from build123d import *

# Parameters (mm, degrees)
F0_W     = 19.05
F0_H     = 50.8
F0_W_2   = 25.4
F0_H_2   = 19.05
F1_DEPTH = 19.05


# Not quite as in the source:
# - a feature names something its author has since deleted; it is built from what else it names


with BuildPart() as f1:
    # F0 (on Top) → F1 (new body)
    with BuildSketch(Plane.XY):
        with Locations((-25.5773371266, 60.6874149844)):
            Rectangle(F0_W, F0_H)
        Polygon((-3.3523371266, 111.4874149844), (-16.0523371266, 111.4874149844), (-16.0523371266, 86.0874149844), (-16.0523371266, 35.2874149844), (-16.0523371266, -15.5125850156), (-16.0523371266, -32.8271351755), (-16.0523371266, -66.3125850156), (-16.0523371266, -91.7125850156), (-3.3523371266, -91.7125850156), (22.0476628734, -91.7125850156), (47.4476628734, -91.7125850156), (72.8476628734, -91.7125850156), (85.5476628734, -91.7125850156), (85.5476628734, -66.3125850156), (85.5476628734, -15.5125850156), (85.5476628734, 35.2874149844), (85.5476628734, 86.0874149844), (85.5476628734, 111.4874149844), (72.8476628734, 111.4874149844), (47.4476628734, 111.4874149844), (22.0476628734, 111.4874149844), align=None)
        Polygon((-16.0523371266, -32.8271351755), (-16.0523371266, -15.5125850156), (-35.1023371266, -15.5125850156), (-35.1023371266, -66.3125850156), (-16.0523371266, -66.3125850156), align=None)
        with Locations((9.3476628734, -101.2375850156)):
            Rectangle(F0_W_2, F0_H_2)
        with Locations((60.1476628734, -101.2375850156)):
            Rectangle(F0_W_2, F0_H_2)
        with Locations((95.0726628734, -40.9125850156)):
            Rectangle(F0_W, F0_H)
        with Locations((95.0726628734, 60.6874149844)):
            Rectangle(F0_W, F0_H)
        with Locations((60.1476628734, 121.0124149844)):
            Rectangle(F0_W_2, F0_H_2)
        with Locations((9.3476628734, 121.0124149844)):
            Rectangle(F0_W_2, F0_H_2)
    extrude(amount=F1_DEPTH)


solid = f1.part
The listing builds one solid part. Answer for the finished solid, in the listing's coordinates (mm). A direction names the side the tool comes from. Coordinates: 2 decimals unless noted, no trailing zeros. Write each loop counter-clockwise with the first axis right and the second up, starting at its lowest first coordinate (ties: lowest second). Pieces come first, ordered by that corner, then holes. Notation, with made-up numbers: M 2.25,75.25 L 58.25,75.25 A22 cw 58.25,107.25 Z; hole C 64,71 d10. An arc over 180 degrees is marked long. Use one line per item in the form item = value.
Item 1: Find the intervals of material crossed by probe 1 along Y at (x, z) = (-27, 16.5); probe 2 along X at (y, z) = (-70, 1.5); probe 3 along Y at (x, z) = (23.5, 3.75), in increasing order.
Model answer:
probe_1 = -66.31 to -15.51, 35.29 to 86.09
probe_2 = -16.05 to 85.55
probe_3 = -91.71 to 111.49
Item 2: Find section C-C, the plane y = 108.5. Give the vertices of the cut face in (x, z).
Model answer:
outline = M -16.05,0 L 85.55,0 L 85.55,19.05 L -16.05,19.05 Z
Item 3: Given P1, Ø6, axis at x = 32.5, z = 8.5, coming from the +Y side; P2, Ø9.5, axis at x = 40, z = 14.5, coming from the -Y side; P3, Ø8, axis at y = -82.5, z = 5, coming from the -X side, each flat-ended and moving along its own axis, determine where each tip first touches the part or whether it passes through.
Model answer:
P1 = 111.49
P2 = -91.71
P3 = -16.05
Item 4: For faces 4 (the face through (22.048, -101, 9)), 5 (the face through (72.848, -101, 9)), 6 (the face through (79, 111.487, 9)), 7 (the face through (-10, 111.487, 9)), 8 (the face through (-26, -66.313, 9)), determine the directions among +Z, -Z, +X, -X, +Y, -Y from which every point of the face is accessible in a straight line to the end or side of a thin tool.
Model answer:
face_4 = +Z, -Z, -Y
face_5 = +Z, -Z, +X, -Y
face_6 = +Z, -Z, +X, +Y
face_7 = +Z, -Z, -X, +Y
face_8 = +Z, -Z, -X, -Y
Item 5: Find section B-B, the plane x = 80. Give the vertices of the cut face in (y, z), plus the area to 3 significant figures.
Model answer:
outline = M -91.71,0 L 111.49,0 L 111.49,19.05 L -91.71,19.05 Z
area = 3,870 mm2
Item 6: Find section A-A, the plane y = -94. Give the vertices of the cut face in (x, z).
Model answer:
outline = M -3.35,0 L 22.05,0 L 22.05,19.05 L -3.35,19.05 Z; M 47.45,0 L 72.85,0 L 72.85,19.05 L 47.45,19.05 Z
Item 7: The mould has two halves that part along X. Classify faces 1 (the face through (-16.052, -79, 9)), 2 (the face through (47.448, -101, 9)), 3 (the face through (-25, -15.513, 9)): released by +X, released by -X, zero draft, split by the parting line, or undercut.
Model answer:
face_1 = released by -X
face_2 = undercut
face_3 = zero draft
